For this review, take the finished solid that the model builds, in its own axes (mm). A direction names the side the tool comes from. Round coordinates to 2 decimals unless told otherwise and drop trailing zeros. Order: outer loops, then holes, each group sorted by start corner. A loop starts at its lowest first (then second) coordinate and runs counter-clockwise, first axis right, second up.
from build123d import *

# Parameters (mm, degrees)
SKETCH1_R           = 38.1
BOSS_EXTRUDE1_DEPTH = 12.7
SKETCH2_R           = 6.223
BOSS_EXTRUDE2_DEPTH = 25.4
SKETCH3_R           = 1.5875
CUT_EXTRUDE1_DEPTH  = 60.56828015
CIRPATTERN1_COUNT   = 4


with BuildPart() as part:
    # Sketch1 → Boss-Extrude1 (new body)
    with BuildSketch(Plane(origin=(0, 0, 0), x_dir=(1, 0, 0), z_dir=(0, 1, 0))):
        with Locations(Location((0, 0, 0), (0, 0, 270))):
            Circle(SKETCH1_R)
    extrude(amount=BOSS_EXTRUDE1_DEPTH)

    # Sketch2 → Boss-Extrude2 (add)
    with BuildSketch(Plane(origin=(0, 12.7, 0), x_dir=(1, 0, 0), z_dir=(0, 1, 0))):
        with Locations(Location((0, 0, 0), (0, 0, 270))):
            Circle(SKETCH2_R)
    extrude(amount=BOSS_EXTRUDE2_DEPTH)

    # Sketch3 → Cut-Extrude1 (cut, through all)
    with BuildSketch(Plane(origin=(0, 12.7, 0), x_dir=(1, 0, 0), z_dir=(0, 1, 0))):
        with Locations(Location((0, 31.75, 0), (0, 0, 270))):
            Circle(SKETCH3_R)
    cut_extrude1 = extrude(amount=-CUT_EXTRUDE1_DEPTH, mode=Mode.SUBTRACT)

    # CirPattern1: Cut-Extrude1 ×4 about axis
    cirpattern1_axis = Axis((0, 0, 0), (0, 1, 0))
    for i in range(1, CIRPATTERN1_COUNT):
        add(cut_extrude1.rotate(cirpattern1_axis, i * 360 / CIRPATTERN1_COUNT), mode=Mode.SUBTRACT)


solid = part.part
(1) Add section A-A on z = 0. Give the boundary of the cut face in (x, y), plus the area to 3 significant figures.
(2) Clearance check with flat-ended pins moving along their axes: P1, Ø2, axis at x = -28.5, y = 11, coming from the +Z side; P2, Ø4, axis at x = 4, y = 22, coming from the -Z side; P3, Ø5, axis at y = 26.5, z = -6.5, coming from the +X side. State where each tip first meets the part, or that it passes through.
(3) Draft analysis for pull direction X (two halves, no side actions). For faces 1 (the face through (-23.183, 6.261, -30.235)), 2 (the face through (0, 38.1, 0)), 3 (the face through (-0.477, 6.439, 30.236)), state which applies: pulls with the +X half, pulls with the -X half, needs draft (parallel to the pull), parting line crosses it, or undercut.
(4) Wall thickness on L1, parallel to Y at x = 31, z = 8; L2, parallel to Z at x = 31.75, y = 7; L3, parallel to X at y = 11.5, z = 31: over which ranges is each line inside the solid? List them lowest first.
(5) Add section D-D on z = 31.75. Give the boundary of the cut face in (x, y), plus the area to 3 significant figures.
(6) Tool access review of faces 4 (the face through (-6.075, 25.222, -1.349)), 5 (the face through (-30.236, 6.439, -0.477)): name each direction out of +Z, -Z, +X, -X, +Y, -Y from which nothing blocks a thin tool from reaching the whole face with its end or side.
(7) Add section C-C on y = 2. Count the separate pieces of the cut face and the enclosed holes in it, plus the area to 3 significant figures.
(8) Add section B-B on x = 0. Give the boundary of the cut face in (y, z), plus the area to 3 significant figures.
Here are the results:
1. outline: (-38.1, 0) - (-33.34, 0) - (-33.34, 12.7) - (-38.1, 12.7) - close; (-30.16, 0) - (30.16, 0) - (30.16, 12.7) - (6.22, 12.7) - (6.22, 38.1) - (-6.22, 38.1) - (-6.22, 12.7) - (-30.16, 12.7) - close; (33.34, 0) - (38.1, 0) - (38.1, 12.7) - (33.34, 12.7) - close
1. area: 1,200 mm2
2. P1: stops at z = 26.37
2. P2: stops at z = -5.89
2. P3: stops at x = 4.77
3. face 1: parting line crosses it
3. face 2: needs draft
3. face 3: undercut
4. L1: y = 0 to 12.7
4. L2: z = -21.06 to -1.59, 1.59 to 21.06
4. L3: x = -22.15 to -1.4, 1.4 to 22.15
5. outline: (-21.06, 0) - (-1.59, 0) - (-1.59, 12.7) - (-21.06, 12.7) - close; (1.59, 0) - (21.06, 0) - (21.06, 12.7) - (1.59, 12.7) - close
5. area: 495 mm2
6. face 4: +Y
6. face 5: +Y, -Y
7. separate pieces: 1
7. enclosed holes: 4
7. area: 4,530 mm2
8. outline: (0, -38.1) - (12.7, -38.1) - (12.7, -33.34) - (0, -33.34) - close; (0, -30.16) - (12.7, -30.16) - (12.7, -6.22) - (38.1, -6.22) - (38.1, 6.22) - (12.7, 6.22) - (12.7, 30.16) - (0, 30.16) - close; (0, 33.34) - (12.7, 33.34) - (12.7, 38.1) - (0, 38.1) - close
8. area: 1,200 mm2
